Part model, mm, in its own coordinate system. Face numbers are marked on the shaded views. A direction names the side the tool comes from. Round coordinates to 2 decimals unless told otherwise and drop trailing zeros. Write each loop counter-clockwise with the first axis right and the second up, starting at its lowest first coordinate (ties: lowest second). Pieces come first, ordered by that corner, then holes. Notation, with made-up numbers: M 88.25,-21 L 98.25,-21 A19 cw 98.25,6 Z; hole C 15.5,19.5 d6. An arc over 180 degrees is marked long. One line per question, with ' | ' between items. Start each with the question number.
1) Mould opens along Y. For the marked faces 1, 2 and 3 say: pulls with the +Y half, pulls with the -Y half, needs draft (parallel to the pull), parting line crosses it, or undercut.
2) Saw through at C-C (y = -17.5). Give the number of separate pieces and of enclosed holes in the cut face, plus the area to 3 significant figures.
3) Saw through at B-B (y = -35). List the corners of the cut face in (x, z), plus the area to 3 significant figures.
4) Saw through at A-A (x = 0). List the corners of the cut face in (y, z).
5) Drop flat-ended pins along their axis: pin 1 Ø4.5 at (x, y) = (0, -35) entering from +Z; pin 2 Ø3 at (y, z) = (-13, 3) entering from +X; pin 3 Ø1.5 at (x, z) = (6.5, 7.5) entering from -Y. Give the stop position or say it passes through.
6) Tool access for the marked faces 4, 5 and 6: list every direction of +Z, -Z, +X, -X, +Y, -Y with a clear straight run to the whole face (end or side of a thin tool).
7) Wall check: probe 1 along Y at (x, z) = (-9, 5.15) (3 decimals); probe 2 along Y at (x, z) = (-9, 9.55) (3 decimals); probe 3 along X at (y, z) = (-19.5, 12.75). Give the ranges that are in metal, low to high. Write a range as [from, to].
```python
from build123d import *
from OCP.BRepFilletAPI import BRepFilletAPI_MakeChamfer

# Parameters (mm, degrees)
SKETCH1_R               = 1.65
SKETCH1_R_2             = 4.475
BOSS_EXTRUDE1_DEPTH     = 20
CHAMFER1_SIZE           = 1
CHAMFER2_SIZE           = 3
CHAMFER2_SIZE2          = 0.528980942
CUT_EXTRUDE1_DEPTH      = 3
CUT_EXTRUDE1_DEPTH_BACK = 3
SKETCH5_R               = 5.475
CHAMFER3_SIZE           = 1


with BuildPart() as part:
    # Sketch1 → Boss-Extrude1 (new body)
    with BuildSketch(Plane.XY):
        with BuildLine():
            ThreePointArc((5.396692576, -1.672784876), (0, 5.65), (-5.396692576, -1.672784876))
            ThreePointArc((-5.396692576, -1.672784876), (-4.701973782, -4.118237099), (-4.124302136, -6.593952399))
            ThreePointArc((-4.124302136, -6.593952399), (-4.919523181, -9.306745557), (-7.616470373, -10.154152821))
            ThreePointArc((-7.616470373, -10.154152821), (-16.475, -17.5), (-7.616470373, -24.845847179))
            ThreePointArc((-7.616470373, -24.845847179), (-4.919523181, -25.693254443), (-4.124302136, -28.406047601))
            ThreePointArc((-4.124302136, -28.406047601), (-4.701973782, -30.881762901), (-5.396692576, -33.327215124))
            ThreePointArc((-5.396692576, -33.327215124), (0, -40.65), (5.396692576, -33.327215124))
            ThreePointArc((5.396692576, -33.327215124), (4.701973782, -30.881762901), (4.124302136, -28.406047601))
            ThreePointArc((4.124302136, -28.406047601), (4.919523181, -25.693254443), (7.616470373, -24.845847179))
            ThreePointArc((7.616470373, -24.845847179), (16.475, -17.5), (7.616470373, -10.154152821))
            ThreePointArc((7.616470373, -10.154152821), (4.919523181, -9.306745557), (4.124302136, -6.593952399))
            ThreePointArc((4.124302136, -6.593952399), (4.701973782, -4.118237099), (5.396692576, -1.672784876))
        make_face()
        Circle(SKETCH1_R, mode=Mode.SUBTRACT)
        with Locations((0, -35)):
            Circle(SKETCH1_R, mode=Mode.SUBTRACT)
        with Locations((9, -17.5)):
            Circle(SKETCH1_R_2, mode=Mode.SUBTRACT)
        with Locations((-9, -17.5)):
            Circle(SKETCH1_R_2, mode=Mode.SUBTRACT)
    extrude(amount=BOSS_EXTRUDE1_DEPTH)

    # Chamfer1
    chamfer1_edges = [part.edges().sort_by_distance(p)[0] for p in [
        (0, -40.65, 0),
        (-4.701973782, -30.881762901, 0),
        (16.475, -17.5, 20),
        (-4.919523181, -25.693254443, 0),
        (-16.475, -17.5, 0),
        (-4.919523181, -9.306745557, 0),
        (-4.701973782, -4.118237099, 0),
        (0, 5.65, 0),
        (4.701973782, -4.118237099, 0),
        (4.919523181, -9.306745557, 0),
        (16.475, -17.5, 0),
        (4.919523181, -25.693254443, 0),
        (4.701973782, -30.881762901, 0),
        (4.919523181, -9.306745557, 20),
        (4.701973782, -4.118237099, 20),
        (0, 5.65, 20),
        (-4.701973782, -4.118237099, 20),
        (-1.65, 0, 0),
        (-1.65, 0, 20),
        (-4.919523181, -9.306745557, 20),
        (-1.65, -35, 0),
        (-1.65, -35, 20),
        (-16.475, -17.5, 20),
        (-4.919523181, -25.693254443, 20),
        (-4.701973782, -30.881762901, 20),
        (0, -40.65, 20),
        (4.701973782, -30.881762901, 20),
        (4.919523181, -25.693254443, 20),
    ]]
    chamfer(chamfer1_edges, length=CHAMFER1_SIZE)

    # Chamfer2: one chamfer whose edges measure the first distance from different faces: ONE call of the kernel's chamfer builder (chamfer() names one face for all edges)
    chamfer2_edges_1 = [part.edges().sort_by_distance(p)[0] for p in [
        (4.525, -17.5, 0),
        (4.525, -17.5, 20),
    ]]
    chamfer2_side_1 = [part.faces().sort_by_distance(p)[0] for p in [
        (4.525, -17.5, 10),
    ]]
    chamfer2_edges_2 = [part.edges().sort_by_distance(p)[0] for p in [
        (-13.475, -17.5, 0),
        (-13.475, -17.5, 20),
    ]]
    chamfer2_side_2 = [part.faces().sort_by_distance(p)[0] for p in [
        (-13.475, -17.5, 10),
    ]]
    chamfer2 = BRepFilletAPI_MakeChamfer(part.part.solid().wrapped)
    for e in chamfer2_edges_1:
        chamfer2.Add(CHAMFER2_SIZE, CHAMFER2_SIZE2, e.wrapped, chamfer2_side_1[0].wrapped)  # the first distance lies on this face
    for e in chamfer2_edges_2:
        chamfer2.Add(CHAMFER2_SIZE, CHAMFER2_SIZE2, e.wrapped, chamfer2_side_2[0].wrapped)  # the first distance lies on this face
    add(Compound.cast(chamfer2.Shape()), mode=Mode.REPLACE)

    # Sketch5 → Cut-Extrude1 (cut, two sides: drawn at the far end of the back side and taken through both)
    with BuildSketch(Plane.XY.offset(10).offset(-CUT_EXTRUDE1_DEPTH_BACK)):
        with Locations((-9, -17.5)):
            Circle(SKETCH5_R)
        with Locations((9, -17.5)):
            Circle(SKETCH5_R)
    extrude(amount=CUT_EXTRUDE1_DEPTH + CUT_EXTRUDE1_DEPTH_BACK, mode=Mode.SUBTRACT)

    # Chamfer3
    chamfer3_edges = [part.edges().sort_by_distance(p)[0] for p in [
        (-13.475, -17.5, 13),
        (-13.475, -17.5, 7),
        (4.525, -17.5, 13),
        (4.525, -17.5, 7),
    ]]
    chamfer(chamfer3_edges, length=CHAMFER3_SIZE - 0.0001)  # a hair under: the kernel refuses the full size


solid = part.part
```
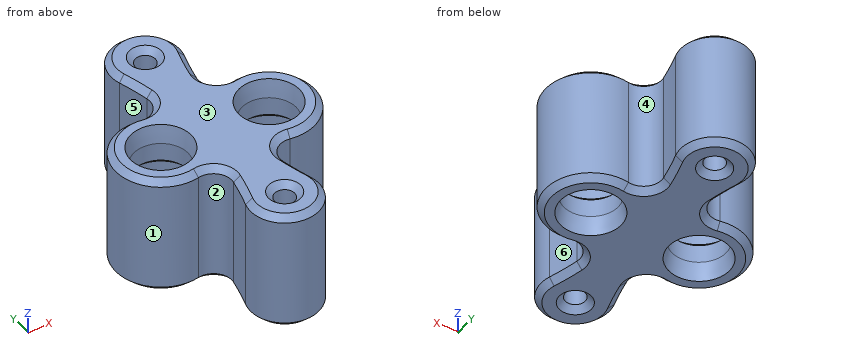
Answer key:
1) face 1: parting line crosses it | face 2: undercut | face 3: needs draft
2) separate pieces: 3 | enclosed holes: 0 | area: 265 mm2
3) outline: M -5.65,1 L -4.65,0 L -2.65,0 L -1.65,1 L -1.65,19 L -2.65,20 L -4.65,20 L -5.65,19 Z; M 1.65,1 L 2.65,0 L 4.65,0 L 5.65,1 L 5.65,19 L 4.65,20 L 2.65,20 L 1.65,19 Z | area: 156 mm2
4) outline: M -40.65,1 L -39.65,0 L -37.65,0 L -36.65,1 L -36.65,19 L -37.65,20 L -39.65,20 L -40.65,19 Z; M -33.35,1 L -32.35,0 L -2.65,0 L -1.65,1 L -1.65,19 L -2.65,20 L -32.35,20 L -33.35,19 Z; M 1.65,1 L 2.65,0 L 4.65,0 L 5.65,1 L 5.65,19 L 4.65,20 L 2.65,20 L 1.65,19 Z
5) pin 1: stops at z = 19.6 | pin 2: stops at x = 15.85 | pin 3: stops at y = -25.1
6) face 4: +Z, -Z | face 5: +Z, -Z, -X | face 6: +Z, -Z, +X
7) probe 1: y = [-24.975, -21.975], [-13.025, -10.025] | probe 2: y = [-24.975, -22.975], [-12.025, -10.025] | probe 3: x = [-16.2, -14.1], [-3.9, 3.9], [14.1, 16.2]
